```python
from build123d import *

# Parameters (mm, degrees)
SKETCH_1_W                  = 15
SKETCH_1_H                  = 15
SKETCH_1_W_2                = 12
SKETCH_1_H_2                = 12
EXTRUDE_1_DEPTH             = 500
SKETCH_2_R                  = 2.25
CUT_EXTRUDE_1_DEPTH         = 25
SKETCH_4_R                  = 2.25
CUT_EXTRUDE_3_DEPTH         = 20
SKETCH_5_R                  = 5
CUT_EXTRUDE_4_DEPTH         = 3.3
SKETCH_6_R                  = 5
CUT_EXTRUDE_5_DEPTH         = 3.3
HOLE_WIZARD_5_4_5_4_1_D     = 5.4
HOLE_WIZARD_10_0_10_1_D     = 10
HOLE_WIZARD_10_0_10_1_DEPTH = 1.5
HOLE_WIZARD_10_0_10_1_TIP   = 3.004303095


with BuildPart() as part:
    # ｽｹｯﾁ1 → ﾎﾞｽ - 押し出し1 (new body)
    with BuildSketch(Plane.XY):
        Rectangle(SKETCH_1_W, SKETCH_1_H)
        Rectangle(SKETCH_1_W_2, SKETCH_1_H_2, mode=Mode.SUBTRACT)
    extrude(amount=EXTRUDE_1_DEPTH)

    # ｽｹｯﾁ2 → ｶｯﾄ - 押し出し1 (cut)
    with BuildSketch(Plane(origin=(7.5, 0, 0), x_dir=(0, 0, -1), z_dir=(1, 0, 0))):
        with Locations((-492.5, 0)):
            Circle(SKETCH_2_R)
        with Locations((-7.5, 0)):
            Circle(SKETCH_2_R)
        with Locations((-317.5, 0)):
            Circle(SKETCH_2_R)
        with Locations((-182.5, 0)):
            Circle(SKETCH_2_R)
    extrude(amount=-CUT_EXTRUDE_1_DEPTH, mode=Mode.SUBTRACT)

    # ｽｹｯﾁ4 → ｶｯﾄ - 押し出し3 (cut)
    with BuildSketch(Plane(origin=(0, -7.5, 0), x_dir=(-1, 0, 0), z_dir=(0, -1, 0))):
        with Locations((0, -22.5)):
            Circle(SKETCH_4_R)
        with Locations((0, -477.5)):
            Circle(SKETCH_4_R)
    extrude(amount=-CUT_EXTRUDE_3_DEPTH, mode=Mode.SUBTRACT)

    # ｽｹｯﾁ5 → ｶｯﾄ - 押し出し4 (cut)
    with BuildSketch(Plane(origin=(7.5, 0, 0), x_dir=(0, 0, -1), z_dir=(1, 0, 0))):
        with Locations((-492.5, 0)):
            Circle(SKETCH_5_R)
        with Locations((-7.5, 0)):
            Circle(SKETCH_5_R)
        with Locations((-182.5, 0)):
            Circle(SKETCH_5_R)
        with Locations((-317.5, 0)):
            Circle(SKETCH_5_R)
    extrude(amount=-CUT_EXTRUDE_4_DEPTH, mode=Mode.SUBTRACT)

    # ｽｹｯﾁ6 → ｶｯﾄ - 押し出し5 (cut)
    with BuildSketch(Plane(origin=(0, 7.5, 0), x_dir=(1, 0, 0), z_dir=(0, 1, 0))):
        with Locations((0, -22.5)):
            Circle(SKETCH_6_R)
        with Locations((0, -477.5)):
            Circle(SKETCH_6_R)
    extrude(amount=-CUT_EXTRUDE_5_DEPTH, mode=Mode.SUBTRACT)

    # Ø5.4 (5.4) 直径の穴1 (through all)
    with Locations(Plane(origin=(7.5, 0, 0), x_dir=(0, 0, -1), z_dir=(1, 0, 0))):
        with Locations((-347.5, 0), (-212.5, 0), (-167.5, 0), (-42.5, 0), (-373.5, 0), (-408.5, 0)):
            Hole(HOLE_WIZARD_5_4_5_4_1_D / 2)

    # Ø10.0 (10) 直径の穴1
    with Locations(Plane.ZY.offset(7.5)):
        with Locations((347.5, 0), (212.5, 0), (167.5, 0), (42.5, 0), (373.5, 0), (408.5, 0)):
            Hole(HOLE_WIZARD_10_0_10_1_D / 2, depth=HOLE_WIZARD_10_0_10_1_DEPTH)
            with Locations((0, 0, -(HOLE_WIZARD_10_0_10_1_DEPTH + HOLE_WIZARD_10_0_10_1_TIP / 2))):  # 118° drill point
                Cone(0, HOLE_WIZARD_10_0_10_1_D / 2, HOLE_WIZARD_10_0_10_1_TIP, mode=Mode.SUBTRACT)


solid = part.part
```
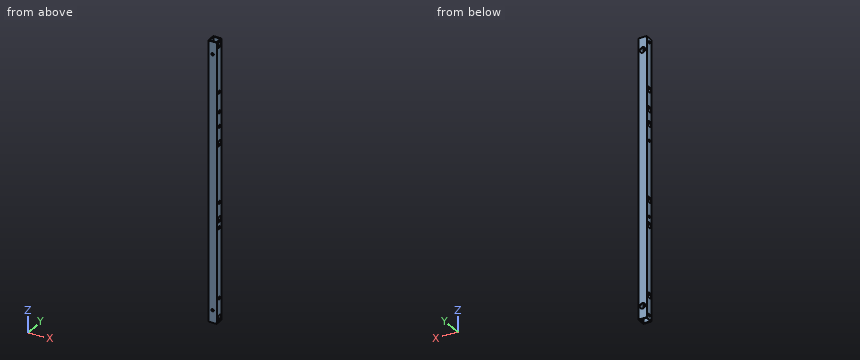
Geometry check sheet. Reference: the model listing, model coordinates, mm. Coordinates: 2 decimals unless noted, no trailing zeros. Write each loop counter-clockwise with the first axis right and the second up, starting at its lowest first coordinate (ties: lowest second). Pieces come first, ordered by that corner, then holes. Notation, with made-up numbers: M 87,50.25 L 108,50.25 A34 ccw 108,82.25 Z; hole C 77.5,-38.75 d2. An arc over 180 degrees is marked long. Answer as a JSON object with one key per item and string values.
1. Scan lines: L1, parallel to Y at x = 4, z = 332.5; L2, parallel to Y at x = -6.45, z = 7.5. Record each from-to range of solid material in increasing order.
Answers below:
{"L1": "y = -7.5 to -6, 6 to 7.5", "L2": "y = -7.5 to -2.25, 2.25 to 7.5"}
2. Section check B-B, the plane z = 462. Enter the section's corners in (x, y), plus the area to 3 significant figures.
Answers below:
{"outline": "M -7.5,-7.5 L 7.5,-7.5 L 7.5,7.5 L -7.5,7.5 Z; hole M -6,-6 L 6,-6 L 6,6 L -6,6 Z", "area": "81.0 mm²"}
3. Section check A-A, the plane x = 0. Enter the section's corners in (y, z), plus the area to 3 significant figures.
Answers below:
{"outline": "M -7.5,0 L -6,0 L -6,20.25 L -7.5,20.25 Z; M -7.5,24.75 L -6,24.75 L -6,475.25 L -7.5,475.25 Z; M -7.5,479.75 L -6,479.75 L -6,500 L -7.5,500 Z; M 6,0 L 7.5,0 L 7.5,17.5 L 6,17.5 Z; M 6,27.5 L 7.5,27.5 L 7.5,472.5 L 6,472.5 Z; M 6,482.5 L 7.5,482.5 L 7.5,500 L 6,500 Z", "area": "1,460 mm²"}
4. Go/stop test with flat-tipped pins: pin 1 Ø9 at (x, z) = (0, 477.5) entering from +Y; pin 2 Ø4.5 at (y, z) = (0, 212.5) entering from -X; pin 3 Ø6 at (y, z) = (0, 408.5) entering from -X. Record where each tip stops, or that it passes through.
Answers below:
{"pin 1": "stops at y = -6", "pin 2": "passes through", "pin 3": "stops at x = 6"}
